```python
from build123d import *

# Parameters (mm, degrees)
SKETCH_1_W          = 14
SKETCH_1_H          = 4
SKETCH_1_W_2        = 145
SKETCH_1_H_2        = 68
EXTRUDE_1_DEPTH     = 4
SKETCH_2_R          = 1.5
CUT_EXTRUDE_1_DEPTH = 4
SKETCH_3_R          = 1.5
SKETCH_3_W          = 4.2
SKETCH_3_H          = 12
CUT_EXTRUDE_2_DEPTH = 10
CUT_EXTRUDE_3_DEPTH = 5
FILLET_1_R          = 3
FILLET_2_R          = 3


with BuildPart() as part:
    # 草图1 → 凸台-拉伸1 (new body)
    with BuildSketch(Plane(origin=(0, 0, 0), x_dir=(1, 0, 0), z_dir=(0, 1, 0))):
        with Locations((-55, -36)):
            Rectangle(SKETCH_1_W, SKETCH_1_H)
        Rectangle(SKETCH_1_W_2, SKETCH_1_H_2)
        with Locations((0, -36)):
            Rectangle(SKETCH_1_W, SKETCH_1_H)
        with Locations((55, -36)):
            Rectangle(SKETCH_1_W, SKETCH_1_H)
        with Locations((-55, 36)):
            Rectangle(SKETCH_1_W, SKETCH_1_H)
        with Locations((55, 36)):
            Rectangle(SKETCH_1_W, SKETCH_1_H)
        with Locations((0, 36)):
            Rectangle(SKETCH_1_W, SKETCH_1_H)
    extrude(amount=EXTRUDE_1_DEPTH)

    # 草图2 → 切除-拉伸1 (cut)
    with BuildSketch(Plane(origin=(0, 4, 0), x_dir=(1, 0, 0), z_dir=(0, 1, 0))):
        with Locations((-63.5, 34)):
            Circle(SKETCH_2_R)
        with Locations((-46.5, 34)):
            Circle(SKETCH_2_R)
        with Locations((-8.5, 34)):
            Circle(SKETCH_2_R)
        with Locations((-63.5, -34)):
            Circle(SKETCH_2_R)
        with Locations((-46.5, -34)):
            Circle(SKETCH_2_R)
        with Locations((-8.5, -34)):
            Circle(SKETCH_2_R)
        with Locations((8.5, 34)):
            Circle(SKETCH_2_R)
        with Locations((46.5, 34)):
            Circle(SKETCH_2_R)
        with Locations((46.5, -34)):
            Circle(SKETCH_2_R)
        with Locations((8.5, -34)):
            Circle(SKETCH_2_R)
        with Locations((63.5, -34)):
            Circle(SKETCH_2_R)
        with Locations((63.5, 34)):
            Circle(SKETCH_2_R)
    extrude(amount=-CUT_EXTRUDE_1_DEPTH, mode=Mode.SUBTRACT)

    # 草图3 → 切除-拉伸2 (cut)
    with BuildSketch(Plane(origin=(0, 4, 0), x_dir=(1, 0, 0), z_dir=(0, 1, 0))):
        with Locations((68.6, 10.5)):
            Circle(SKETCH_3_R)
        with Locations((68.6, 19.5)):
            Circle(SKETCH_3_R)
        with Locations((64.4, 19.5)):
            Circle(SKETCH_3_R)
        with Locations((64.4, 10.5)):
            Circle(SKETCH_3_R)
        with Locations((66.5, 15)):
            Rectangle(SKETCH_3_W, SKETCH_3_H)
        with BuildLine():
            ThreePointArc((65.9, 10.5), (65.460660172, 11.560660172), (64.4, 12))
            Line((64.4, 12), (64.4, 9))
            ThreePointArc((64.4, 9), (65.460660172, 9.439339828), (65.9, 10.5))
        make_face()
        with BuildLine():
            Line((64.4, 9), (64.4, 12))
            ThreePointArc((64.4, 12), (62.9, 10.5), (64.4, 9))
        make_face()
        with BuildLine():
            ThreePointArc((65.9, 19.5), (65.460660172, 20.560660172), (64.4, 21))
            Line((64.4, 21), (64.4, 18))
            ThreePointArc((64.4, 18), (65.460660172, 18.439339828), (65.9, 19.5))
        make_face()
        with BuildLine():
            Line((64.4, 18), (64.4, 21))
            ThreePointArc((64.4, 21), (62.9, 19.5), (64.4, 18))
        make_face()
        with BuildLine():
            ThreePointArc((70.1, 19.5), (69.660660172, 20.560660172), (68.6, 21))
            Line((68.6, 21), (68.6, 18))
            ThreePointArc((68.6, 18), (69.660660172, 18.439339828), (70.1, 19.5))
        make_face()
        with BuildLine():
            Line((68.6, 18), (68.6, 21))
            ThreePointArc((68.6, 21), (67.1, 19.5), (68.6, 18))
        make_face()
        with BuildLine():
            ThreePointArc((70.1, 10.5), (69.660660172, 11.560660172), (68.6, 12))
            Line((68.6, 12), (68.6, 9))
            ThreePointArc((68.6, 9), (69.660660172, 9.439339828), (70.1, 10.5))
        make_face()
        with BuildLine():
            Line((68.6, 9), (68.6, 12))
            ThreePointArc((68.6, 12), (67.1, 10.5), (68.6, 9))
        make_face()
        with BuildLine():
            ThreePointArc((64.4, -18), (62.9, -19.5), (64.4, -21))
            Line((64.4, -21), (64.4, -18))
        make_face()
        with BuildLine():
            Line((64.4, -18), (64.4, -21))
            ThreePointArc((64.4, -21), (65.460660172, -20.560660172), (65.9, -19.5))
            ThreePointArc((65.9, -19.5), (65.460660172, -18.439339828), (64.4, -18))
        make_face()
        with Locations((64.4, -19.5)):
            Circle(SKETCH_3_R)
        with Locations((68.6, -19.5)):
            Circle(SKETCH_3_R)
        with Locations((68.6, -10.5)):
            Circle(SKETCH_3_R)
        with Locations((64.4, -10.5)):
            Circle(SKETCH_3_R)
        with Locations((66.5, -15)):
            Rectangle(SKETCH_3_W, SKETCH_3_H)
        with BuildLine():
            ThreePointArc((68.6, -18), (67.1, -19.5), (68.6, -21))
            Line((68.6, -21), (68.6, -18))
        make_face()
        with BuildLine():
            Line((68.6, -18), (68.6, -21))
            ThreePointArc((68.6, -21), (69.660660172, -20.560660172), (70.1, -19.5))
            ThreePointArc((70.1, -19.5), (69.660660172, -18.439339828), (68.6, -18))
        make_face()
        with BuildLine():
            ThreePointArc((64.4, -9), (62.9, -10.5), (64.4, -12))
            Line((64.4, -12), (64.4, -9))
        make_face()
        with BuildLine():
            Line((64.4, -9), (64.4, -12))
            ThreePointArc((64.4, -12), (65.460660172, -11.560660172), (65.9, -10.5))
            ThreePointArc((65.9, -10.5), (65.460660172, -9.439339828), (64.4, -9))
        make_face()
        with BuildLine():
            ThreePointArc((68.6, -9), (67.1, -10.5), (68.6, -12))
            Line((68.6, -12), (68.6, -9))
        make_face()
        with BuildLine():
            Line((68.6, -9), (68.6, -12))
            ThreePointArc((68.6, -12), (69.660660172, -11.560660172), (70.1, -10.5))
            ThreePointArc((70.1, -10.5), (69.660660172, -9.439339828), (68.6, -9))
        make_face()
    cut_extrude_2 = extrude(amount=-CUT_EXTRUDE_2_DEPTH, mode=Mode.SUBTRACT)

    # 镜向1: 切除-拉伸2 across plane
    add(cut_extrude_2.mirror(Plane(origin=(0, 0, 0), x_dir=(0, 0, 1), z_dir=(1, 0, 0))), mode=Mode.SUBTRACT)

    # 草图4 → 切除-拉伸3 (cut)
    with BuildSketch(Plane(origin=(0, 4, 0), x_dir=(1, 0, 0), z_dir=(0, 1, 0))):
        Polygon((-33.989694233, 0), (-56, 19.809275191), (-56, -19.809275191), align=None)
        Polygon((-8.989694233, 22.5), (-53.010305767, 22.5), (-31, 2.690724809), align=None)
        Polygon((-6, 19.809275191), (-28.010305767, 0), (-6, -19.809275191), align=None)
        Polygon((-8.989694233, -22.5), (-31, -2.690724809), (-53.010305767, -22.5), align=None)
        Polygon((28.010305767, 0), (6, 19.809275191), (6, -19.809275191), align=None)
        Polygon((8.989694233, 22.5), (31, 2.690724809), (53.010305767, 22.5), align=None)
        Polygon((56, 19.809275191), (33.989694233, 0), (56, -19.809275191), align=None)
        Polygon((53.010305767, -22.5), (31, -2.690724809), (8.989694233, -22.5), align=None)
    extrude(amount=-CUT_EXTRUDE_3_DEPTH, mode=Mode.SUBTRACT)

    # 圆角1
    fillet_1_edges = [part.edges().sort_by_distance(p)[0] for p in [
        (6, 2, -19.809275191),
        (28.010305767, 2, 0),
        (6, 2, 19.809275191),
        (-31, 2, 2.690724809),
        (-8.989694233, 2, 22.5),
        (-53.010305767, 2, 22.5),
        (-8.989694233, 2, -22.5),
        (-31, 2, -2.690724809),
        (-53.010305767, 2, -22.5),
        (-6, 2, -19.809275191),
        (-6, 2, 19.809275191),
        (-28.010305767, 2, 0),
        (53.010305767, 2, 22.5),
        (8.989694233, 2, 22.5),
        (31, 2, 2.690724809),
        (53.010305767, 2, -22.5),
        (31, 2, -2.690724809),
        (8.989694233, 2, -22.5),
        (56, 2, -19.809275191),
        (56, 2, 19.809275191),
        (33.989694233, 2, 0),
        (-33.989694233, 2, 0),
        (-56, 2, 19.809275191),
        (-56, 2, -19.809275191),
    ]]
    fillet(fillet_1_edges, radius=FILLET_1_R)

    # 圆角2
    fillet_2_edges = [part.edges().sort_by_distance(p)[0] for p in [
        (-72.5, 2, 34),
        (-72.5, 2, -34),
        (72.5, 2, -34),
        (72.5, 2, 34),
    ]]
    fillet(fillet_2_edges, radius=FILLET_2_R)


solid = part.part
```
Work out the finished part from the listing and answer in its coordinate system (mm). A direction names the side the tool comes from. Coordinates: 2 decimals unless noted, no trailing zeros. Loops run counter-clockwise (first coordinate to the right, second up) from the corner with the lowest first, then second, coordinate; pieces in that order, holes last. Notation, with made-up numbers: (-14, 87.5) - (28, 87.5) arc R4 cw to (28, 92.5) - close; hole circle Ø2 at (85, -35.75). An arc over 180 degrees is marked (long way). Use a Markdown table: item, result.
Item 1: Consider probe 1 along Z at (x, y) = (66, 3.45); probe 2 along Z at (x, y) = (55, 0.95); probe 3 along X at (y, z) = (2.3, -22). Determine where each line is inside the solid, lowest interval first. Write a range as from..to.
Evaluation:
| item | result |
|---|---|
| probe 1 | z = -34..-21, -9..9, 21..34 |
| probe 2 | z = -38..-15.31, 15.31..38 |
| probe 3 | x = -72.5..-46.85, -15.15..15.15, 46.85..72.5 |
Item 2: The mould has two halves that part along Z. Classify faces 1 (the cylindrical face through (-63.5, 2, -32.5)), 2 (the cylindrical face through (-70.1, 2, 10.5)), 3 (the flat face through (7, 2, -36)): +Z half, -Z half, draft (parallel to the pull), parting line (faces both ways), or undercut.
Evaluation:
| item | result |
|---|---|
| face 1 | -Z half |
| face 2 | undercut |
| face 3 | draft |
Item 3: Find section A-A, the plane z = -19.5. Determine the outline of the cut face in (x, y), and give its area (3 significant figures).
Evaluation:
| item | result |
|---|---|
| outline | (-72.5, 0) - (-70.1, 0) - (-70.1, 4) - (-72.5, 4) - close; (-62.9, 0) - (-48.19, 0) - (-48.19, 4) - (-62.9, 4) - close; (-13.81, 0) - (13.81, 0) - (13.81, 4) - (-13.81, 4) - close; (48.19, 0) - (62.9, 0) - (62.9, 4) - (48.19, 4) - close; (70.1, 0) - (72.5, 0) - (72.5, 4) - (70.1, 4) - close |
| area | 247 mm2 |
Item 4: Find section B-B, the plane x = -8.5. Determine the outline of the cut face in (y, z), and give its area (3 significant figures).
Evaluation:
| item | result |
|---|---|
| outline | (0, -32.5) - (4, -32.5) - (4, -16.03) - (0, -16.03) - close; (0, 16.03) - (4, 16.03) - (4, 32.5) - (0, 32.5) - close |
| area | 132 mm2 |
Item 5: For faces 4 (the flat face through (27, 2, -34)), 5 (the flat face through (-62, 2, 36)), 6 (the flat face through (-64.4, 2, 15)), determine the directions among +Z, -Z, +X, -X, +Y, -Y from which every point of the face is accessible in a straight line to the end or side of a thin tool.
Evaluation:
| item | result |
|---|---|
| face 4 | -Z, +Y, -Y |
| face 5 | +Z, -X, +Y, -Y |
| face 6 | +Y, -Y |
Item 6: Given pin 1 Ø1.2 at (y, z) = (2, -37) entering from -X; pin 2 Ø2 at (y, z) = (2.5, 36.5) entering from +X; pin 3 Ø2 at (x, y) = (-66, 1) entering from -Z, each flat-ended and moving along its own axis, determine where each tip first touches the part or whether it passes through.
Evaluation:
| item | result |
|---|---|
| pin 1 | stops at x = -62 |
| pin 2 | stops at x = 62 |
| pin 3 | stops at z = -34 |
Item 7: Find section C-C, the plane y = 1. State how many separate pieces and enclosed holes the cut face has, and give its area (3 significant figures).
Evaluation:
| item | result |
|---|---|
| separate pieces | 1 |
| enclosed holes | 12 |
| area | 6,600 mm2 |
